The model under review builds one solid part; all positions refer to its coordinate system, in mm. Coordinates: 2 decimals unless noted, no trailing zeros. Write each loop counter-clockwise with the first axis right and the second up, starting at its lowest first coordinate (ties: lowest second). Pieces come first, ordered by that corner, then holes. Notation, with made-up numbers: (63, 6.5) - (72, 6.5) arc R13 cw to (72, 27.5) - close; hole circle Ø4 at (-18, -14.75). An arc over 180 degrees is marked (long way). Put each result on its own line as item: value.
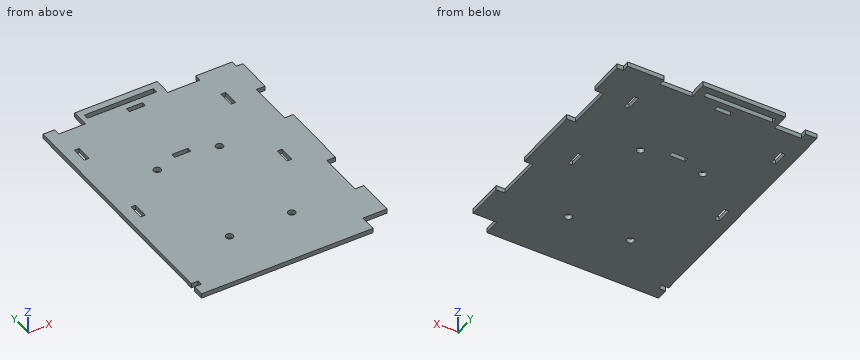
from build123d import *

# Parameters (mm, degrees)
AUFSATZ_LINEAR_AUSTRAGEN1_DEPTH = 2
SKIZZE2_R                       = 1.6
SKIZZE2_W                       = 2
SKIZZE2_H                       = 7
SKIZZE2_W_2                     = 7
SKIZZE2_H_2                     = 2
SCHNITT_LINEAR_AUSTRAGEN1_DEPTH = 2
SKIZZE3_W                       = 30.2
SKIZZE3_H                       = 2.2
SCHNITT_LINEAR_AUSTRAGEN2_DEPTH = 2


with BuildPart() as part:
    # Skizze1 → Aufsatz-Linear austragen1 (new body)
    with BuildSketch(Plane.XY):
        Polygon((39.278745883, -130.531139266), (-35.721254117, -130.531139266), (-35.721254117, -125.531139266), (-32.721254117, -125.531139266), (-32.721254117, -123.331139266), (-35.721254117, -123.331139266), (-35.721254117, -18.031139266), (-30.721254117, -18.031139266), (-30.721254117, -21.031139266), (-28.689548947, -21.031139266), (-23.428125466, -21.031139266), (-18.990357652, -21.031139266), (-18.990357652, -13.331139266), (17.009642348, -13.331139266), (17.009642348, -21.031139266), (22.500868798, -21.031139266), (28.500868798, -21.031139266), (31.045701771, -21.031139266), (31.045701771, -18.031139266), (47.045701771, -18.031139266), (47.045701771, -21.031139266), (49.778745883, -21.031139266), (49.778745883, -36.831139266), (45.978745883, -36.831139266), (45.978745883, -56.831139266), (49.778745883, -56.831139266), (49.778745883, -86.831139266), (45.978745883, -86.831139266), (45.978745883, -106.831139266), (49.778745883, -106.831139266), (49.778745883, -123.331139266), (39.278745883, -123.331139266), align=None)
    extrude(amount=AUFSATZ_LINEAR_AUSTRAGEN1_DEPTH)

    # Skizze2 → Schnitt-Linear austragen1 (cut)
    with BuildSketch(Plane.XY.offset(2)):
        with Locations((-10.721254117, -58.531139266)):
            Circle(SKIZZE2_R)
        with Locations((16.478745883, -58.531139266)):
            Circle(SKIZZE2_R)
        with Locations((-8.721254117, -106.531139266)):
            Circle(SKIZZE2_R)
        with Locations((18.478745883, -106.531139266)):
            Circle(SKIZZE2_R)
        with Locations((-29.721254117, -35.831139266)):
            Rectangle(SKIZZE2_W, SKIZZE2_H)
        with Locations((34.278745883, -35.831139266)):
            Rectangle(SKIZZE2_W, SKIZZE2_H)
        with Locations((-29.721254117, -75.831139266)):
            Rectangle(SKIZZE2_W, SKIZZE2_H)
        with Locations((34.278745883, -75.831139266)):
            Rectangle(SKIZZE2_W, SKIZZE2_H)
        with Locations((2.278745883, -54.531139266)):
            Rectangle(SKIZZE2_W_2, SKIZZE2_H_2)
        with Locations((2.278745883, -22.331139266)):
            Rectangle(SKIZZE2_W_2, SKIZZE2_H_2)
    extrude(amount=-SCHNITT_LINEAR_AUSTRAGEN1_DEPTH, mode=Mode.SUBTRACT)

    # Skizze3 → Schnitt-Linear austragen2 (cut)
    with BuildSketch(Plane.XY.offset(2)):
        with Locations((-1.561818921, -17.431139266)):
            Rectangle(SKIZZE3_W, SKIZZE3_H)
    extrude(amount=-SCHNITT_LINEAR_AUSTRAGEN2_DEPTH, mode=Mode.SUBTRACT)


solid = part.part
1. Consider section D-D on x = -21. State the section outline as (y, z) points, plus the area to 3 significant figures.
Determined:
outline: (-130.53, 0) - (-21.03, 0) - (-21.03, 2) - (-130.53, 2) - close
area: 219 mm^2
2. Consider section A-A on x = 11. State the section outline as (y, z) points, plus the area to 3 significant figures.
Determined:
outline: (-130.53, 0) - (-18.53, 0) - (-18.53, 2) - (-130.53, 2) - close; (-16.33, 0) - (-13.33, 0) - (-13.33, 2) - (-16.33, 2) - close
area: 230 mm^2
3. To check wall thickness, follow probe 1 along X at (y, z) = (-20, 0.45); probe 2 along X at (y, z) = (-106.5, 1.2); probe 3 along Y at (x, z) = (3.5, 1.25). State the ranges of each line that lie inside material, in increasing order.
Determined:
probe 1: x = -35.72 to -30.72, -18.99 to 17.01, 31.05 to 47.05
probe 2: x = -35.72 to -10.32, -7.12 to 16.88, 20.08 to 45.98
probe 3: y = -130.53 to -55.53, -53.53 to -23.33, -21.33 to -18.53, -16.33 to -13.33
4. Consider section C-C on z = 1.35. Give the number of separate pieces and of enclosed holes in the cut face, plus the area to 3 significant figures.
Determined:
separate pieces: 1
enclosed holes: 11
area: 9,290 mm^2
5. Consider section B-B on y = -91. State the section outline as (x, z) points.
Determined:
outline: (-35.72, 0) - (45.98, 0) - (45.98, 2) - (-35.72, 2) - close
6. For pin 1 Ø1 at (x, z) = (-23.5, 1) entering from +Y, flat-tipped, find the tip position at first contact; note if it passes through.
Determined:
pin 1: stops at y = -21.03
